Autodesk Fusion 360 part; units mm, degrees
sketch "Boceto1" plane through (0, 0, 0) normal (1, 0, 0) x (0, 1, 0)
  line L0 (0, 0) -> (0, 35)
  line L1 (0, 35) -> (35, 35)
  line L2 (35, 35) -> (35, 0)
  line L3 (35, 0) -> (0, 0)
  dimension "d1" = 35
  dimension "d2" = 35
extrude "Extruir1" add sketch "Boceto1" along normal blind 19
sketch "Boceto2" plane through (19, 0, 0) normal (1, 0, 0) x (0, 1, 0)
  line L0 (35, 0) -> (35, 35)
  line L1 (35, 35) -> (0, 35)
  line L2 (0, 35) -> (0, 0)
  line L3 (0, 0) -> (35, 0)
  circle A0 centre (17.5, 17.5) radius 8.5
  dimension "d5" = 17
extrude "Extruir2" cut sketch "Boceto2" against normal blind 15 contours A0
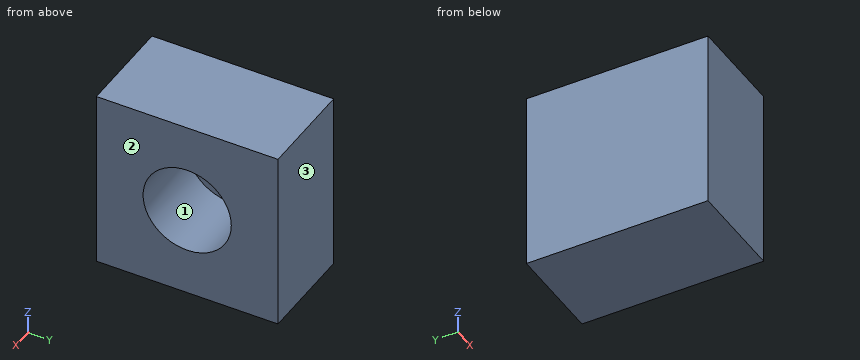
CAD build for the part. Positions are in the model's coordinates, mm. Face numbers are marked on the shaded views. Round coordinates to 2 decimals unless told otherwise and drop trailing zeros. Loops run counter-clockwise (first coordinate to the right, second up) from the corner with the lowest first, then second, coordinate; pieces in that order, holes last.
(1) Cut at B-B (x = 7.5). Give the cut face in (y, z), plus the area to 3 significant figures.
(2) Drop flat-ended pins along their axis: pin 1 (5 mm diameter, centred on x = 9.5, z = 11, fed in from -Y); pin 2 (1 mm diameter, centred on y = 19.5, z = 19, fed in from +X). Give the stop position or say it passes through.
(3) Wall check: line 1 along Z through (x, y) = (14.75, 17.5); line 2 along X through (y, z) = (15.5, 23); line 3 along Z through (x, y) = (10, 23). Give the ranges that are in metal, low to high.
(4) Cut at A-A (y = 17.5). Give the cut face in (x, z), plus the area to 3 significant figures.
(5) Two-plate mould, pull along Y, no slides. Class the marked faces 1, 2 and 3: +Y half, -Y half, draft (parallel to the pull), parting line (faces both ways), or undercut.
Findings below:
1. outline: (0, 0) - (35, 0) - (35, 35) - (0, 35) - close; hole circle Ø17 at (17.5, 17.5)
1. area: 998 mm2
2. pin 1: stops at y = 0
2. pin 2: stops at x = 4
3. line 1: z = 0 to 9, 26 to 35
3. line 2: x = 0 to 4
3. line 3: z = 0 to 11.02, 23.98 to 35
4. outline: (0, 0) - (19, 0) - (19, 9) - (4, 9) - (4, 26) - (19, 26) - (19, 35) - (0, 35) - close
4. area: 410 mm2
5. face 1: undercut
5. face 2: draft
5. face 3: +Y half
